from build123d import *

# Parameters (mm, degrees)
EXTRUDE_1_DEPTH              = 3
CUT_EXTRUDE_1_REACH          = 104.025
SKETCH_2_W                   = 5
SKETCH_2_H                   = 10
HOLE_WIZARD_M2_1_D           = 2.4
HOLE_WIZARD_M2_1_CBORE_D     = 4.4
HOLE_WIZARD_M2_1_CBORE_DEPTH = 2
CUT_EXTRUDE_2_REACH          = 104.025
SKETCH_5_R                   = 4
HOLE_WIZARD_M2_2_D           = 2.4
HOLE_WIZARD_M2_2_CBORE_D     = 4.4
HOLE_WIZARD_M2_2_CBORE_DEPTH = 2
HOLE_WIZARD_M2_3_D           = 2.4
HOLE_WIZARD_M2_3_CBORE_D     = 4.4
HOLE_WIZARD_M2_3_CBORE_DEPTH = 2
CUT_EXTRUDE_3_DEPTH          = 3
HOLE_WIZARD_M2_5_D           = 2.4
HOLE_WIZARD_M2_5_CBORE_D     = 4.4
HOLE_WIZARD_M2_5_CBORE_DEPTH = 2
HOLE_WIZARD_M2_6_D           = 2.4
HOLE_WIZARD_M2_6_CBORE_D     = 4.4
HOLE_WIZARD_M2_6_CBORE_DEPTH = 2
SKETCH_17_OUTSIDE_W          = 82.796
SKETCH_17_OUTSIDE_H          = 242.796
CUT_EXTRUDE_4_DEPTH          = 10


with BuildPart() as part:
    # 草图1 → 凸台-拉伸1 (new body)
    with BuildSketch(Plane.XY):
        Polygon((20, 5), (20, 45), (19.258297735, 54.944681764), (13.241702265, 95.055318236), (7.5, 100), (-7.5, 100), (-13.241702265, 95.055318236), (-19.258297735, 54.944681764), (-20, 45), (-20, 5), (-19.379826327, -4.961389384), (-7.748069469, -98.015444247), (-5.5, -100), (5.5, -100), (7.748069469, -98.015444247), (19.379826327, -4.961389384), align=None)
    extrude(amount=EXTRUDE_1_DEPTH)

    # 草图2 → 切除-拉伸1 (cut, up to next)
    with BuildSketch(Plane.XY.offset(3), mode=Mode.PRIVATE) as cut_extrude_1_sk1:
        Polygon((10, -5), (-10, -5), (0, -22.320508076), align=None)
    cut_extrude_1_tool1 = extrude(cut_extrude_1_sk1.sketch, amount=-CUT_EXTRUDE_1_REACH, mode=Mode.PRIVATE) & part.part
    # 草图2 → 切除-拉伸1 (cut, up to next)
    with BuildSketch(Plane.XY.offset(3), mode=Mode.PRIVATE) as cut_extrude_1_sk2:
        Polygon((6.211088907, -70), (13.938881842, -8.177656525), (2.5, -27.990381057), (2.5, -70), align=None)
    cut_extrude_1_tool2 = extrude(cut_extrude_1_sk2.sketch, amount=-CUT_EXTRUDE_1_REACH, mode=Mode.PRIVATE) & part.part
    # 草图2 → 切除-拉伸1 (cut, up to next)
    with BuildSketch(Plane.XY.offset(3), mode=Mode.PRIVATE) as cut_extrude_1_sk3:
        Polygon((-13.938881842, -8.177656525), (-2.5, -27.990381057), (-2.5, -70), (-6.211088907, -70), align=None)
    cut_extrude_1_tool3 = extrude(cut_extrude_1_sk3.sketch, amount=-CUT_EXTRUDE_1_REACH, mode=Mode.PRIVATE) & part.part
    # 草图2 → 切除-拉伸1 (cut, up to next)
    with BuildSketch(Plane.XY.offset(3), mode=Mode.PRIVATE) as cut_extrude_1_sk4:
        with Locations((0, -85)):
            Rectangle(SKETCH_2_W, SKETCH_2_H)
    cut_extrude_1_tool4 = extrude(cut_extrude_1_sk4.sketch, amount=-CUT_EXTRUDE_1_REACH, mode=Mode.PRIVATE) & part.part
    add(cut_extrude_1_tool1.solids().sort_by_distance((0, -10.773503, 3))[0], mode=Mode.SUBTRACT)
    add(cut_extrude_1_tool2.solids().sort_by_distance((6.712708, -39.914502, 3))[0], mode=Mode.SUBTRACT)
    add(cut_extrude_1_tool3.solids().sort_by_distance((-6.712708, -39.914502, 3))[0], mode=Mode.SUBTRACT)
    add(cut_extrude_1_tool4.solids().sort_by_distance((0, -85, 3))[0], mode=Mode.SUBTRACT)

    # M2 凹头盖螺钉的柱形沉头孔1 (through all)
    with Locations(Plane(origin=(5.586088907, -75, 0), x_dir=(-1, 0, 0), z_dir=(0, 0, -1))):
        with Locations((0, 0), (11.172177814, 0)):
            CounterBoreHole(HOLE_WIZARD_M2_1_D / 2, HOLE_WIZARD_M2_1_CBORE_D / 2, HOLE_WIZARD_M2_1_CBORE_DEPTH)

    # 草图5 → 切除-拉伸2 (cut, up to next)
    with BuildSketch(Plane(origin=(0, 0, 0), x_dir=(-1, 0, 0), z_dir=(0, 0, -1)), mode=Mode.PRIVATE) as cut_extrude_2_sk1:
        with Locations((0, 25)):
            Circle(SKETCH_5_R)
    cut_extrude_2_tool1 = extrude(cut_extrude_2_sk1.sketch, amount=-CUT_EXTRUDE_2_REACH, mode=Mode.PRIVATE) & part.part
    add(cut_extrude_2_tool1.solids().sort_by_distance((0, 25, 0))[0], mode=Mode.SUBTRACT)

    # M2 凹头盖螺钉的柱形沉头孔2 (through all)
    with Locations(Plane(origin=(8, 25, 0), x_dir=(-1, 0, 0), z_dir=(0, 0, -1))):
        with Locations((0, 0), (8, 8), (16, 0), (8, -8)):
            CounterBoreHole(HOLE_WIZARD_M2_2_D / 2, HOLE_WIZARD_M2_2_CBORE_D / 2, HOLE_WIZARD_M2_2_CBORE_DEPTH)

    # M2 凹头盖螺钉的柱形沉头孔3 (through all)
    with Locations(Plane(origin=(12.880020708, -5.011657807, 0), x_dir=(-1, 0, 0), z_dir=(0, 0, -1))):
        with Locations((0, 0), (25.760041416, 0)):
            CounterBoreHole(HOLE_WIZARD_M2_3_D / 2, HOLE_WIZARD_M2_3_CBORE_D / 2, HOLE_WIZARD_M2_3_CBORE_DEPTH)

    # 草图10 → 切除-拉伸3 (cut)
    with BuildSketch(Plane(origin=(0, 0, 0), x_dir=(-1, 0, 0), z_dir=(0, 0, -1))):
        Polygon((-14.016935065, 56.180852205), (-10.679274874, 78.431920145), (-8.411945476, 80.068406675), (-4.470648492, 79.385634325), (-2.5, 77.04424815), (-2.5, 56.2029795), (-4.5, 54.2029795), (-12.313615971, 54.2029795), align=None)
        Polygon((-9.344020618, 87.333615184), (-8.2970205, 94.313615971), (0, 94.313615971), (8.2970205, 94.313615971), (9.344020618, 87.333615184), (7.670053032, 85.014356303), (0, 83.685631227), (-7.670053032, 85.014356303), align=None)
        Polygon((4.5, 54.2029795), (12.313615971, 54.2029795), (14.016935065, 56.180852205), (10.679274874, 78.431920145), (8.411945476, 80.068406675), (4.470648492, 79.385634325), (2.5, 77.04424815), (2.5, 56.2029795), align=None)
    extrude(amount=-CUT_EXTRUDE_3_DEPTH, mode=Mode.SUBTRACT)

    # M2 凹头盖螺钉的柱形沉头孔5 (through all)
    with Locations(Plane(origin=(0, 79.840052868, 0), x_dir=(-1, 0, 0), z_dir=(0, 0, -1))):
        with Locations((0, 0)):
            CounterBoreHole(HOLE_WIZARD_M2_5_D / 2, HOLE_WIZARD_M2_5_CBORE_D / 2, HOLE_WIZARD_M2_5_CBORE_DEPTH)

    # M2 凹头盖螺钉的柱形沉头孔6 (through all)
    with Locations(Plane(origin=(12.880020708, 14.988342193, 0), x_dir=(-1, 0, 0), z_dir=(0, 0, -1))):
        with Locations((0, 0), (25.760041416, 0)):
            CounterBoreHole(HOLE_WIZARD_M2_6_D / 2, HOLE_WIZARD_M2_6_CBORE_D / 2, HOLE_WIZARD_M2_6_CBORE_DEPTH)

    # 草图17 outside → 切除-拉伸4 (cut)
    with BuildSketch(Plane(origin=(0, 0, 0), x_dir=(-1, 0, 0), z_dir=(0, 0, -1))):
        Rectangle(SKETCH_17_OUTSIDE_W, SKETCH_17_OUTSIDE_H)
        Polygon((-20, 5), (20, 5), (20, 99.998273705), (7.5, 100), (-7.5, 100), (-20, 99.998273705), align=None, mode=Mode.SUBTRACT)
    extrude(amount=-CUT_EXTRUDE_4_DEPTH, mode=Mode.SUBTRACT)


solid = part.part
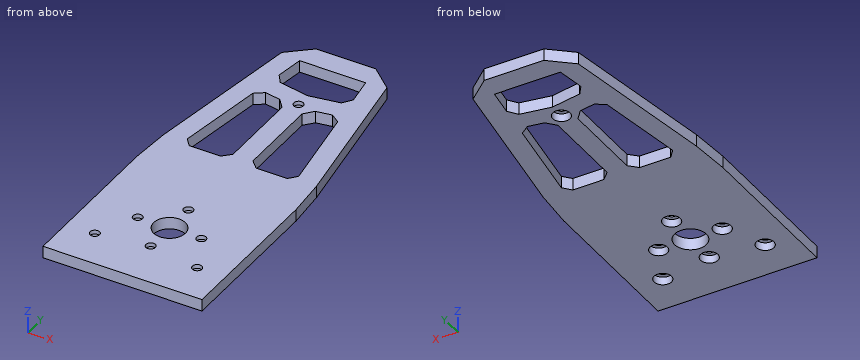
Input: part model. Units: mm. Frame: model coordinates. Round coordinates to 2 decimals unless told otherwise and drop trailing zeros. Loops run counter-clockwise (first coordinate to the right, second up) from the corner with the lowest first, then second, coordinate; pieces in that order, holes last. Notation, with made-up numbers: M 62,-25.75 L 82,-25.75 A16 cw 82,-15.75 Z; hole C 57.25,-15.75 d9. An arc over 180 degrees is marked long. Answer as CSV lines item,"result". Start each with the question number.
(1) First-contact query: pin 1 (1.3 mm diameter, centred on x = 12, y = 14.5, fed in from -Z). Flat tip, straight axial feed; report the tip coordinate or a pass-through.
(2) Section C-C, the plane z = 0.6. State how many separate pieces and enclosed holes the cut face has, plus the area to 3 significant figures.
(3) Section B-B, the plane x = 17. Output: boundary loops of the cut face in (y, z), plus the area to 3 significant figures.
(4) Section D-D, the plane x = -16.5. Output: boundary loops of the cut face in (y, z).
(5) Line query: line 1 (Y direction, x = 0, z = 0.5); line 2 (Y direction, x = -3, z = 2.75); line 3 (X direction, y = 60, z = 1.1). Output: solid intervals per line, ascending. Write a range as [from, to].
(6) Section A-A, the plane y = 25. Output: boundary loops of the cut face in (x, z), plus the area to 3 significant figures.
Values found:
1,pin 1,"stops at z = 2"
2,separate pieces,"1"
2,enclosed holes,"11"
2,area,"2,580 mm²"
3,outline,"M 5,0 L 70,0 L 70,3 L 5,3 Z"
3,area,"195 mm²"
4,outline,"M 5,0 L 73.33,0 L 73.33,3 L 5,3 Z"
5,line 1,"y = [5, 14.8], [19.2, 21], [29, 30.8], [35.2, 77.64], [82.04, 83.69], [94.31, 100]"
5,line 2,"y = [5, 22.35], [27.65, 55.7], [77.64, 84.21], [94.31, 100]"
5,line 3,"x = [-18.5, -13.44], [-2.5, 2.5], [13.44, 18.5]"
6,outline,"M -20,0 L -10.2,0 L -10.2,2 L -9.2,2 L -9.2,3 L -20,3 Z; M -6.8,2 L -5.8,2 L -5.8,0 L -4,0 L -4,3 L -6.8,3 Z; M 4,0 L 5.8,0 L 5.8,2 L 6.8,2 L 6.8,3 L 4,3 Z; M 9.2,2 L 10.2,2 L 10.2,0 L 20,0 L 20,3 L 9.2,3 Z"
6,area,"73.6 mm²"
